Geometry check sheet. Reference: the model listing, model coordinates, mm. Face numbers are marked on the shaded views. A direction names the side the tool comes from. Coordinates: 2 decimals unless noted, no trailing zeros. Order: outer loops, then holes, each group sorted by start corner. A loop starts at its lowest first (then second) coordinate and runs counter-clockwise, first axis right, second up. Notation, with made-up numbers: M 58,58.25 L 85,58.25 A29 cw 85,93.25 Z; hole C -14,81 d4. An arc over 180 degrees is marked long. One line per item, written item: value. Start each with the question number.
1) Go/stop test with flat-tipped pins: P1, Ø18.5, axis at y = 19, z = 12.5, coming from the -X side; P2, Ø4, axis at x = -14.5, z = 16, coming from the +Y side. Record where each tip stops, or that it passes through.
2) Access from +Z, -Z, +X, -X, +Y, -Y to the whole of each face (thin tool, end or side, straight path). Record for the marked faces 4 and 5.
3) Sectioned sample at B-B, the plane y = 30. Enter the section's corners in (x, z), then the cut area to 3 significant figures.
4) Thickness scan on L1, parallel to Y at x = -4.25, z = 20; L2, parallel to X at y = 39, z = 30.5; L3, parallel to Y at x = -10.5, z = 24. Record the ranges inside material, lowest first. Write a range as from..to.
5) Draft check along Y on the marked faces 1, 2 and 3. Enter one of: pulls with the +Y half, pulls with the -Y half, needs draft (parallel to the pull), parting line crosses it, or undercut.
6) Sectioned sample at D-D, the plane z = 29.5. Enter the section's corners in (x, y), then the cut area to 3 significant figures.
7) Sectioned sample at C-C, the plane x = -2.5. Enter the section's corners in (y, z), then the cut area to 3 significant figures.
8) Sectioned sample at A-A, the plane z = 20. Enter the section's corners in (x, y).
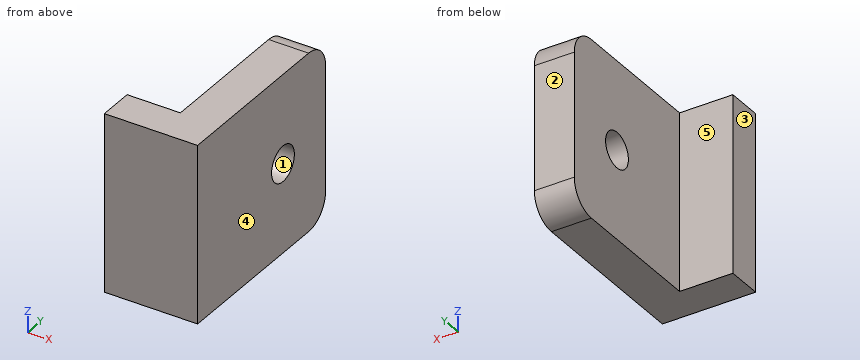
```python
from build123d import *

# Parameters (mm, degrees)
EXTRUDE_1_DEPTH     = 40
FILLET_1_R          = 6
SKETCH_2_R          = 4
CUT_EXTRUDE_1_DEPTH = 62.392181913


with BuildPart() as part:
    # 草图1 → 凸台-拉伸1 (new body)
    with BuildSketch(Plane.XY):
        Polygon((0, 0), (-21, 0), (-21, 8), (-9, 8), (-9, 45), (0, 45), align=None)
    extrude(amount=EXTRUDE_1_DEPTH)

    # 圆角1
    fillet_1_edges = [part.edges().sort_by_distance(p)[0] for p in [
        (-4.5, 45, 40),
        (-4.5, 45, 0),
    ]]
    fillet(fillet_1_edges, radius=FILLET_1_R)

    # 草图2 → 切除-拉伸1 (cut, through all)
    with BuildSketch(Plane.ZY.offset(9)):
        with Locations((20, 30)):
            Circle(SKETCH_2_R)
    extrude(amount=-CUT_EXTRUDE_1_DEPTH, mode=Mode.SUBTRACT)


solid = part.part
```
Final values:
1. P1: stops at x = -9
1. P2: stops at y = 8
2. face 4: +Z, -Z, +X, +Y, -Y
2. face 5: +Z, -Z, -X, +Y
3. outline: M -9,0 L 0,0 L 0,16 L -9,16 Z; M -9,24 L 0,24 L 0,40 L -9,40 Z
3. area: 288 mm^2
4. L1: y = 0..26, 34..45
4. L2: x = -9..0
4. L3: y = 0..8
5. face 1: undercut
5. face 2: pulls with the +Y half
5. face 3: needs draft
6. outline: M -21,0 L 0,0 L 0,45 L -9,45 L -9,8 L -21,8 Z
6. area: 501 mm^2
7. outline: M 0,0 L 39,0 A6 ccw 45,6 L 45,34 A6 ccw 39,40 L 0,40 Z; hole C 30,20 d8
7. area: 1,730 mm^2
8. outline: M -21,0 L 0,0 L 0,26 L -9,26 L -9,8 L -21,8 Z; M -9,34 L 0,34 L 0,45 L -9,45 Z
